Design review of the part built by this model. Coordinates are the model's own, in mm. A direction names the side the tool comes from. Round coordinates to 2 decimals unless told otherwise and drop trailing zeros. Loops run counter-clockwise (first coordinate to the right, second up) from the corner with the lowest first, then second, coordinate; pieces in that order, holes last. Notation, with made-up numbers: M -2,23 L 10,23 A35 cw 10,61 Z; hole C -23,54.25 d1. An arc over 180 degrees is marked long. Use a Markdown table: item, result.
from build123d import *

# Parameters (mm, degrees)
SKETCH1_R           = 49
BOSS_EXTRUDE1_DEPTH = 5
SKETCH2_R           = 4.5
SKETCH2_R_2         = 3
BOSS_EXTRUDE2_DEPTH = 4
SKETCH2_2_R         = 4.5
SKETCH2_2_R_2       = 3
BOSS_EXTRUDE3_DEPTH = 4
SKETCH3_R           = 4
SKETCH3_R_2         = 3.5
BOSS_EXTRUDE4_DEPTH = 3
SKETCH4_R           = 1.5
CUT_EXTRUDE1_DEPTH  = 5
SKETCH5_R           = 1.5
CUT_EXTRUDE2_DEPTH  = 5


with BuildPart() as part:
    # Sketch1 → Boss-Extrude1 (new body)
    with BuildSketch(Plane.XY):
        with Locations((-26.650582962, 0)):
            Circle(SKETCH1_R)
    extrude(amount=BOSS_EXTRUDE1_DEPTH)

    # Sketch2 → Boss-Extrude2 (add)
    with BuildSketch(Plane(origin=(0, 0, 0), x_dir=(-1, 0, 0), z_dir=(0, 0, -1))):
        with Locations((26.650582962, 0)):
            Circle(SKETCH2_R)
        with Locations((26.650582962, 0)):
            Circle(SKETCH2_R_2, mode=Mode.SUBTRACT)
    extrude(amount=-BOSS_EXTRUDE2_DEPTH)

    # Sketch2<2> → Boss-Extrude3 (add)
    with BuildSketch(Plane(origin=(0, 0, 0), x_dir=(-1, 0, 0), z_dir=(0, 0, -1))):
        with Locations((26.650582962, 0)):
            Circle(SKETCH2_2_R)
        with Locations((26.650582962, 0)):
            Circle(SKETCH2_2_R_2, mode=Mode.SUBTRACT)
    extrude(amount=BOSS_EXTRUDE3_DEPTH)

    # Sketch3 → Boss-Extrude4 (add)
    with BuildSketch(Plane.XY.offset(5)):
        with Locations((-26.650582962, 0)):
            Circle(SKETCH3_R)
        with Locations((-26.650582962, 0)):
            Circle(SKETCH3_R_2, mode=Mode.SUBTRACT)
    extrude(amount=BOSS_EXTRUDE4_DEPTH)

    # Sketch4 → Cut-Extrude1 (cut)
    with BuildSketch(Plane.XY.offset(5)):
        with Locations((-26.650582962, 0)):
            Circle(SKETCH4_R)
    extrude(amount=-CUT_EXTRUDE1_DEPTH, mode=Mode.SUBTRACT)

    # Sketch5 → Cut-Extrude2 (cut)
    with BuildSketch(Plane.XY.offset(5)):
        with Locations((-34.650582962, 0)):
            Circle(SKETCH5_R)
        with Locations((-42.650582962, 0)):
            Circle(SKETCH5_R)
        with Locations((-57.150582962, 0)):
            Circle(SKETCH5_R)
        with Locations((-26.650582962, 8)):
            Circle(SKETCH5_R)
        with Locations((-26.650582962, 16)):
            Circle(SKETCH5_R)
        with Locations((-26.650582962, 30.5)):
            Circle(SKETCH5_R)
        with Locations((-18.650582962, 0)):
            Circle(SKETCH5_R)
        with Locations((-10.650582962, 0)):
            Circle(SKETCH5_R)
        with Locations((3.849417038, 0)):
            Circle(SKETCH5_R)
        with Locations((-26.650582962, -8)):
            Circle(SKETCH5_R)
        with Locations((-26.650582962, -16)):
            Circle(SKETCH5_R)
        with Locations((-26.650582962, -30.5)):
            Circle(SKETCH5_R)
    extrude(amount=-CUT_EXTRUDE2_DEPTH, mode=Mode.SUBTRACT)


solid = part.part
1. Take a section at D-D on y = 16. Give the boundary of the cut face in (x, z).
Check values:
| item | result |
|---|---|
| outline | M -72.96,0 L -28.15,0 L -28.15,5 L -72.96,5 Z; M -25.15,0 L 19.66,0 L 19.66,5 L -25.15,5 Z |
2. Take a section at B-B on y = -30.5. Give the boundary of the cut face in (x, z).
Check values:
| item | result |
|---|---|
| outline | M -65,0 L -28.15,0 L -28.15,5 L -65,5 Z; M -25.15,0 L 11.7,0 L 11.7,5 L -25.15,5 Z |
3. The part is to be moulded in two halves that separate along Y. For faces 3 (the face through (-55.72, 0.45, 2.54)), 4 (the face through (-30.647, 0.176, 6.479)), 5 (the face through (-27, -2, 5)), 6 (the face through (-16, 1, 5)), say which applies: pulls with the +Y half, pulls with the -Y half, needs draft (parallel to the pull), parting line crosses it, or undercut.
Check values:
| item | result |
|---|---|
| face 3 | undercut |
| face 4 | parting line crosses it |
| face 5 | undercut |
| face 6 | needs draft |
4. Take a section at A-A on z = 3. Count the separate pieces of the cut face and the enclosed holes in it, and give its area (3 significant figures).
Check values:
| item | result |
|---|---|
| separate pieces | 1 |
| enclosed holes | 13 |
| area | 7,450 mm² |
5. Wall thickness on line 1 along Z through (x, y) = (-25, -33.5); line 2 along X through (y, z) = (-0.5, -2.5); line 3 along X through (y, z) = (42.5, 2.5): over which ranges is each line inside the solid? List them lowest first. Write a range as from..to.
Check values:
| item | result |
|---|---|
| line 1 | z = 0..5 |
| line 2 | x = -31.12..-29.61, -23.69..-22.18 |
| line 3 | x = -51.04..-2.26 |
6. Insertion check: pin 1 (1.8 mm diameter, centred on x = -26.65, y = 30.5, fed in from -Z); pin 2 (4 mm diameter, centred on x = 11.5, y = -30.5, fed in from +Z); pin 3 (5 mm diameter, centred on x = -42.65, y = 0, fed in from -Z); pin 4 (4 mm diameter, centred on x = 10, z = 2, fed in from +Y). Each pin has a flat end and moves straight along its axis. Give the tip position at first contact, or say it passes through.
Check values:
| item | result |
|---|---|
| pin 1 | passes through |
| pin 2 | stops at z = 5 |
| pin 3 | stops at z = 0 |
| pin 4 | stops at y = 34.65 |
7. Machinability: for faces 1 (the face through (-35.841, -0.913, 2.535)), 2 (the face through (-28, -1, 0)), which of the approach directions +Z, -Z, +X, -X, +Y, -Y give a long, thin tool a straight path to every point of the face, cutting with its end or side? Answer none if there is none.
Check values:
| item | result |
|---|---|
| face 1 | +Z, -Z |
| face 2 | -Z |
